```python
from build123d import *

# Parameters (mm, degrees)
FILLET1_R = 10


with BuildPart() as part:
    # Sketch1 → Revolve2 (revolve)
    with BuildSketch(Plane.XY, mode=Mode.PRIVATE) as revolve2_sk:
        with BuildLine():
            Line((-3.59, -36.15), (-3.59, -21.15))
            Line((-3.59, -21.15), (-8, 0))
            Line((-8, 0), (-8.766277994, 9.195335924))
            ThreePointArc((-8.766277994, 9.195335924), (-11.137120078, 17.107504902), (-16.502977942, 23.386906109))
            Line((-16.502977942, 23.386906109), (-22.5, 28))
            Line((-22.5, 28), (-25.5, 28))
            Line((-25.5, 28), (-18.455600302, 22.584866513))
            ThreePointArc((-18.455600302, 22.584866513), (-13.092321233, 16.315659868), (-10.71591345, 8.415001644))
            Line((-10.71591345, 8.415001644), (-10.003752773, 0))
            Line((-10.003752773, 0), (-5.59, -21.15))
            Line((-5.59, -21.15), (-5.59, -36.15))
            ThreePointArc((-5.59, -36.15), (-11.447864376, -50.292135624), (-25.59, -56.15))
            Line((-25.59, -56.15), (-25.59, -58.15))
            Line((-25.59, -58.15), (-35, -58.15))
            Line((-35, -58.15), (-37, -60.15))
            Line((-37, -60.15), (0, -60.15))
            Line((0, -60.15), (0, -58.15))
            Line((0, -58.15), (-3.59, -36.15))
        make_face()
        with BuildLine():
            Line((-16.42484861, -56.15), (-16.42484861, -58.15))
            Line((-16.42484861, -58.15), (-2.026453361, -58.15))
            Line((-2.026453361, -58.15), (-4.561439674, -42.615264931))
            ThreePointArc((-4.561439674, -42.615264931), (-9.045746613, -50.651299247), (-16.42484861, -56.15))
        make_face(mode=Mode.SUBTRACT)
    revolve(revolve2_sk.sketch.rotate(Axis((0, 74.39046888, 0), (0, -1, 0)), 270), axis=Axis((0, 74.39046888, 0), (0, -1, 0)))

    # Fillet1
    # the kernel refuses this fillet: 10 mm, written as the material it takes off along each edge
    with BuildSketch(Plane(origin=(0, -56.15, 0), x_dir=(0, 0, 1), z_dir=(1, 0, 0))) as fillet1_piece_1:
        with BuildLine():
            CenterArc((18.631445006, 9.181818182), FILLET1_R, 283.412011605, 30.683417109)
            Line((25.59, 2), (25.7291711, 1.856363636))
            ThreePointArc((25.7291711, 1.856363636), (25.79, 1), (25.79, 0))
            Line((25.79, 0), (25.59, -0.2))
            ThreePointArc((25.59, -0.2), (23.277858136, -0.335463392), (20.997353704, -0.74))
            Line((20.997353704, -0.74), (20.950963337, -0.545454545))
        make_face()
    revolve(axis=Axis((0, -56.15, 0), (0, -1, 0)), mode=Mode.SUBTRACT)


solid = part.part
```
Can you work these out from the model? Positions are in its coordinate system, mm. A direction names the side the tool comes from. Round coordinates to 2 decimals unless told otherwise and drop trailing zeros. Order: outer loops, then holes, each group sorted by start corner. A loop starts at its lowest first (then second) coordinate and runs counter-clockwise, first axis right, second up.
(1) On a 3-axis mill with a long thin cutter (end or side, diameter ignored), from which of +Z, -Z, +X, -X, +Y, -Y can I reach the whole of each face in a straight line? I mean faces 1 (the face through (3, -58.15, 0)), 2 (the face through (23, 28, 0)), 3 (the face through (26, -58.15, -2)). Say none if no direction works.
Results are:
face 1: none
face 2: +Z, -Z, +X, -X, +Y
face 3: +Y
(2) We'd pull the mould along Y, two halves only. Please class faces 4 (the face through (-1.75, -10.427, 5.557)), 5 (the face through (2.18, -28.54, -2.85)), 6 (the face through (9.994, -57.164, -13.034)): +Y half, -Y half, draft (parallel to the pull), parting line (faces both ways), or undercut.
Results are:
face 4: +Y half
face 5: draft
face 6: undercut
(3) If we section it at A-A (y = 5.5): Please give me the cut outline in (x, z), plus the area to 3 significant figures.
Results are:
outline: circle Ø20.94 at (0, 0); hole circle Ø16.92 at (0, 0)
area: 120 mm2
